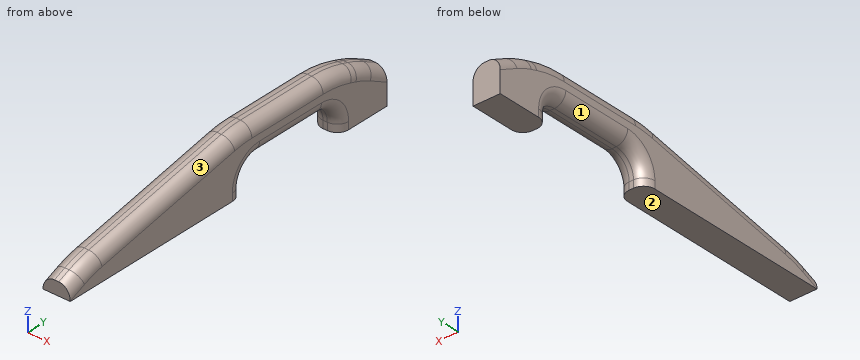
from build123d import *

# Parameters (mm, degrees)
F1_DEPTH      = 15.08125
F1_DEPTH_BACK = 15.08125
F2_R          = 127
F3_R          = 22.225
F4_R          = 12.7


with BuildPart() as f1:
    # F0 (on Right) → F1 (new body, two sides)
    with BuildSketch(Plane.YZ) as f1_sk:
        Polygon((0, 14.2875), (0, 0), (220.6625, 0), (220.6625, 30.48), (344.4875, 30.48), (344.4875, 0), (406.4, 0), (406.4, 38.1), (381, 51.60542), (344.4875, 63.5), (220.6625, 63.5), (25.4, 25.06916), align=None)
    extrude(amount=F1_DEPTH)
    extrude(f1_sk.sketch, amount=-F1_DEPTH_BACK)

    # F2
    f2_edges = [f1.edges().sort_by_distance(p)[0] for p in [
        (0, 25.4, 25.06916),
        (0, 381, 51.60542),
        (0, 344.4875, 63.5),
        (0, 220.6625, 63.5),
    ]]
    fillet(f2_edges, radius=F2_R)

    # F3
    f3_edges = [f1.edges().sort_by_distance(p)[0] for p in [
        (0, 220.6625, 30.48),
        (0, 344.4875, 30.48),
    ]]
    fillet(f3_edges, radius=F3_R)

    # F4
    f4_edges = [f1.edges().sort_by_distance(p)[0] for p in [
        (15.08125, 282.575, 30.48),
        (15.08125, 278.682185, 63.5),
        (-15.08125, 278.682185, 63.5),
        (-15.08125, 282.575, 30.48),
    ]]
    fillet(f4_edges, radius=F4_R)


solid = f1.part
Input: part model. Units: mm. Frame: model coordinates. Face numbers are marked on the shaded views. Coordinates: 2 decimals unless noted, no trailing zeros. Loops run counter-clockwise (first coordinate to the right, second up) from the corner with the lowest first, then second, coordinate; pieces in that order, holes last.
(1) Section B-B on x = -6. Return the cut outline in (y, z) (1 decimal), then the cut area to 3 significant figures.
(2) Material intervals for probe 1 along Z at (x, y) = (-6.5, 212.5); probe 2 along Y at (x, z) = (9.5, 7); probe 3 along Y at (x, z) = (6.5, 4.5), sorted ascending.
(3) Pull-direction query (Y, two-part tool) for the marked faces 1, 2 and 3; classes: released by +Y, released by -Y, zero draft, split by the parting line, or undercut.
(4) Section A-A on y = 316. Return the cut outline in (x, z), then the cut area to 3 significant figures.
(5) First-contact query: pin 1 Ø2.5 at (x, y) = (0, 298) entering from -Z; pin 2 Ø12 at (x, y) = (3.5, 358) entering from +Z; pin 3 Ø8 at (y, z) = (339.5, 11) entering from -X; pin 4 Ø12 at (y, z) = (177.5, 55.5) entering from -X. Flat tips, straight axial feed; report the tip coordinate or a pass-through.
Data:
1. outline: (0, 0) - (220.1, 0) - (220.1, 8.3) arc R22.8 cw to (242.9, 31) - (322.3, 31) arc R22.8 cw to (345, 8.3) - (345, 0) - (406.4, 0) - (406.4, 37.5) - (390.5, 45.9) arc R126.5 ccw to (370.3, 54.5) - (363.5, 56.8) arc R126.5 ccw to (324.3, 63) - (233, 63) arc R126.5 ccw to (208.6, 60.6) - (38.5, 27.1) arc R126.5 ccw to (13.5, 19.4) - (0, 13.7) - close
1. area: 16,300 mm2
2. probe 1: z = 0 to 61.13
2. probe 2: y = 0 to 218.48, 346.67 to 406.4
2. probe 3: y = 0 to 219.98, 345.17 to 406.4
3. face 1: undercut
3. face 2: zero draft
3. face 3: released by -Y
4. outline: (-15.08, 43.18) arc R12.7 ccw to (-2.38, 30.48) - (2.38, 30.48) arc R12.7 ccw to (15.08, 43.18) - (15.08, 50.8) arc R12.7 ccw to (2.38, 63.5) - (-2.38, 63.5) arc R12.7 ccw to (-15.08, 50.8) - close
4. area: 858 mm2
5. pin 1: stops at z = 30.48
5. pin 2: stops at z = 60.43
5. pin 3: passes through
5. pin 4: stops at x = -12.85
